```python
from build123d import *

# Parameters (mm, degrees)
BOSS_EXTRUDE1_DEPTH = 7.5
SKETCH3_R           = 16.5
BOSS_EXTRUDE2_DEPTH = 2.5
SKETCH7_R           = 5
BOSS_EXTRUDE3_DEPTH = 10
BOSS_EXTRUDE4_DEPTH = 5


with BuildPart() as part:
    # Sketch1 → Boss-Extrude1 (new body, symmetric)
    with BuildSketch(Plane.XY):
        with BuildLine():
            Line((-81.983854392, -19.771263634), (88.350129521, -14.621102291))
            ThreePointArc((88.350129521, -14.621102291), (99.92815548, 1.466347152), (85.441176471, 14.993510707))
            Line((85.441176471, 14.993510707), (-84.411764706, 19.991347609))
            ThreePointArc((-84.411764706, 19.991347609), (-104.962820533, -1.218932468), (-81.983854392, -19.771263634))
        make_face()
    extrude(amount=BOSS_EXTRUDE1_DEPTH, both=True)

    # Sketch3 → Boss-Extrude2 (add, symmetric)
    with BuildSketch(Plane.XY.offset(7.5)):
        with Locations((-85, 0)):
            Circle(SKETCH3_R)
    extrude(amount=BOSS_EXTRUDE2_DEPTH, both=True)

    # Sketch7 → Boss-Extrude3 (add)
    with BuildSketch(Plane(origin=(0, 0, -7.5), x_dir=(-1, 0, 0), z_dir=(0, 0, -1))):
        with Locations((85, 0)):
            Circle(SKETCH7_R)
    extrude(amount=BOSS_EXTRUDE3_DEPTH)

    # Sketch12 → Boss-Extrude4 (add, symmetric)
    with BuildSketch(Plane(origin=(0, 0, 0), x_dir=(1, 0, 0), z_dir=(0, 1, 0))):
        with BuildLine():
            ThreePointArc((103.475564721, 23.657260108), (81.077385627, -0.642858818), (104.760808967, -23.692146559))
            ThreePointArc((104.760808967, -23.692146559), (106.947065998, -21.505889528), (104.760808967, -19.319632497))
            ThreePointArc((104.760808967, -19.319632497), (85.448289772, -0.524215738), (103.712763513, 19.291184529))
            ThreePointArc((103.712763513, 19.291184529), (106.436573923, 21.628643871), (103.475564721, 23.657260108))
        make_face()
    extrude(amount=BOSS_EXTRUDE4_DEPTH, both=True)


solid = part.part
```
Model file for the job. Use its own axes, mm. A direction names the side the tool comes from. Give positions to 0.01 mm unless a question says otherwise; leave off trailing zeros. Loops run counter-clockwise (first coordinate to the right, second up) from the corner with the lowest first, then second, coordinate; pieces in that order, holes last. Notation, with made-up numbers: M 89,62.25 L 103,62.25 A29 ccw 103,88.25 Z; hole C 87.25,52 d1. An arc over 180 degrees is marked long. Use one line per item in the form item = value.
Item 1: Which spindle directions (+Z, -Z, +X, -X, +Y, -Y) get a long thin tool onto all of the face, cutting with end or side? Do faces 4 (the flat face through (-85, 0, -17.5)), 5 (the cylindrical face through (90.553, 0.07, -18.959)), 6 (the cylindrical face through (-97.16, 11.15, 8.77)), 7 (the flat face through (-85, 0, 10)), 8 (the cylindrical face through (-89.619, -1.915, -12.43)). Say none if no direction does.
Filled in:
face_4 = -Z, -X, +Y, -Y
face_5 = -Z, +Y, -Y
face_6 = +Z
face_7 = +Z, -X, +Y, -Y
face_8 = -Z
Item 2: Slice it at C-C on x = -61. List the corners of the cut face in (y, z), and give its area (3 significant figures).
Filled in:
outline = M -19.14,-7.5 L 19.3,-7.5 L 19.3,7.5 L -19.14,7.5 Z
area = 577 mm^2
Item 3: Slice it at D-D on y = -12.5. List the corners of the cut face in (x, z), and give its area (3 significant figures).
Filled in:
outline = M -100.61,-7.5 L 93.29,-7.5 L 93.29,7.5 L -74.23,7.5 L -74.23,10 L -95.77,10 L -95.77,7.5 L -100.61,7.5 Z
area = 2,960 mm^2
Item 4: Slice it at B-B on z = 5. List the corners of the cut face in (x, y), and give its area (3 significant figures).
Filled in:
outline = M -84.41,19.99 A20 ccw long -81.98,-19.77 L 88.35,-14.62 A15 ccw 85.44,14.99 Z
area = 6,900 mm^2
Item 5: Flat gauge pins, fed straight in: pin 1 Ø10 at (x, y) = (-75, -6) entering from +Z; pin 2 Ø4 at (y, z) = (-11, -1) entering from +X; pin 3 Ø12 at (x, y) = (-28.5, 4.5) entering from +Z; pin 4 Ø8 at (x, z) = (96, 12) entering from -Y (3 decimals). Where does each tip first touch, or does it go through?
Filled in:
pin_1 = 10
pin_2 = 97
pin_3 = 7.5
pin_4 = through
Item 6: Slice it at A-A on y = 0. List the corners of the cut face in (x, z), and give its area (3 significant figures).
Filled in:
outline = M -105,-7.5 L -90,-7.5 L -90,-17.5 L -80,-17.5 L -80,-7.5 L 82.29,-7.5 A23.69 ccw 103.48,-23.66 A2.26 ccw long 103.71,-19.29 A19.32 cw 86.96,-7.5 L 100,-7.5 L 100,7.5 L 86.96,7.5 A19.32 cw 104.76,19.32 A2.19 ccw 104.76,23.69 A23.69 ccw 82.29,7.5 L -68.5,7.5 L -68.5,10 L -101.5,10 L -101.5,7.5 L -105,7.5 Z
area = 3,500 mm^2
Item 7: Drill centre lines: L1, parallel to Z at x = -11, y = -2; L2, parallel to Z at x = 90, y = 1; L3, parallel to Y at x = 93, z = -15.5. Where is each one in solid material? Low to high.
Filled in:
L1 = -7.5 to 7.5
L2 = -18.53 to -12.46, -7.5 to 7.5, 12.46 to 18.53
L3 = -5 to 5
Item 8: Two-plate mould, pull along X, no slides. Class faces 1 (the cylindrical face through (99.955, 1.164, 0.105)), 2 (the flat face through (-4, 0, -7.5)), 3 (the flat face through (93, -5, -16)): released by +X, released by -X, zero draft, split by the parting line, or undercut.
Filled in:
face_1 = released by +X
face_2 = undercut
face_3 = zero draft
